```python
from build123d import *

# Parameters (mm, degrees)
BOSS_EXTRUDE1_DEPTH = 28.575
CUT_EXTRUDE1_REACH  = 35.651
SKETCH2_R           = 1.5
CUT_EXTRUDE2_REACH  = 35.651
SKETCH3_R           = 1.5
FILLET1_R           = 2.54


with BuildPart() as part:
    # Sketch1 → Boss-Extrude1 (new body)
    with BuildSketch(Plane.XY):
        Polygon((-1.3335, 11.523094809), (-3.365093559, 11.563734809), (-3.596414524, 0), (3.596414524, 0), (3.365093559, 11.563734809), (1.3335, 11.523094809), (1.524, 2), (-1.524, 2), align=None)
        Polygon((-1.23825, 16.284642214), (-1.3335, 11.523094809), (-3.365093559, 11.563734809), (-3.269843559, 16.325282214), align=None)
    extrude(amount=BOSS_EXTRUDE1_DEPTH)

    # Sketch2 → Cut-Extrude1 (cut, up to next)
    with BuildSketch(Plane(origin=(3.594975959, 0.071913903, 0), x_dir=(0, 0, -1), z_dir=(0.9997999799959991, 0.01999999999999963, 0)), mode=Mode.PRIVATE) as cut_extrude1_sk1:
        with Locations(Location((-23.8125, 8.31911996, 0), (0, 0, 90))):
            Circle(SKETCH2_R)
    cut_extrude1_tool1 = extrude(cut_extrude1_sk1.sketch, amount=-CUT_EXTRUDE1_REACH, mode=Mode.PRIVATE) & part.part
    # Sketch2 → Cut-Extrude1 (cut, up to next)
    with BuildSketch(Plane(origin=(3.594975959, 0.071913903, 0), x_dir=(0, 0, -1), z_dir=(0.9997999799959991, 0.01999999999999963, 0)), mode=Mode.PRIVATE) as cut_extrude1_sk2:
        with Locations(Location((-4.7625, 8.31911996, 0), (0, 0, 90))):
            Circle(SKETCH2_R)
    cut_extrude1_tool2 = extrude(cut_extrude1_sk2.sketch, amount=-CUT_EXTRUDE1_REACH, mode=Mode.PRIVATE) & part.part
    add(cut_extrude1_tool1.solids().sort_by_distance((3.428594, 8.38937, 23.8125))[0], mode=Mode.SUBTRACT)
    add(cut_extrude1_tool2.solids().sort_by_distance((3.428594, 8.38937, 4.7625))[0], mode=Mode.SUBTRACT)

    # Sketch3 → Cut-Extrude2 (cut, up to next)
    with BuildSketch(Plane(origin=(-3.594975959, 0.071913903, 0), x_dir=(0, 0, 1), z_dir=(-0.9997999799959991, 0.019999999999999622, 0)), mode=Mode.PRIVATE) as cut_extrude2_sk1:
        with Locations(Location((4.7625, 8.29879996, 0), (0, 0, 270))):
            Circle(SKETCH3_R)
    cut_extrude2_tool1 = extrude(cut_extrude2_sk1.sketch, amount=-CUT_EXTRUDE2_REACH, mode=Mode.PRIVATE) & part.part
    # Sketch3 → Cut-Extrude2 (cut, up to next)
    with BuildSketch(Plane(origin=(-3.594975959, 0.071913903, 0), x_dir=(0, 0, 1), z_dir=(-0.9997999799959991, 0.019999999999999622, 0)), mode=Mode.PRIVATE) as cut_extrude2_sk2:
        with Locations(Location((23.8125, 8.29879996, 0), (0, 0, 270))):
            Circle(SKETCH3_R)
    cut_extrude2_tool2 = extrude(cut_extrude2_sk2.sketch, amount=-CUT_EXTRUDE2_REACH, mode=Mode.PRIVATE) & part.part
    add(cut_extrude2_tool1.solids().sort_by_distance((-3.429, 8.369054, 4.7625))[0], mode=Mode.SUBTRACT)
    add(cut_extrude2_tool2.solids().sort_by_distance((-3.429, 8.369054, 23.8125))[0], mode=Mode.SUBTRACT)

    # Fillet1
    # the kernel refuses this fillet: 2.54 mm, written as the material it takes off along each edge
    with BuildSketch(Plane(origin=(1.3335, 11.523094809, -6.221703947), x_dir=(0.9997999799960309, 0.019999999998416385, 0), z_dir=(0, 0, 1))) as fillet1_piece_1:
        with BuildLine():
            CenterArc((2.54, -2.488681579), FILLET1_R, 101.536959033, 78.463040967)
            Line((0, -2.488681579), (-0.0508, -2.488681579))
            Line((-0.0508, -2.488681579), (-0.0508, 0))
            Line((-0.0508, 0), (0, 0.0508))
            ThreePointArc((0, 0.0508), (1.016, 0.0508), (2.02184, 0.049773632))
            Line((2.02184, 0.049773632), (2.032, 0))
        make_face()
    extrude(amount=41.018407893, mode=Mode.SUBTRACT)
    with BuildSketch(Plane(origin=(-1.23825, 16.284642214, -6.221703947), x_dir=(-0.9997999799960307, 0.019999999998425156, 0), z_dir=(0, 0, 1))) as fillet1_piece_2:
        with BuildLine():
            CenterArc((2.54, 2.488681579), FILLET1_R, 180, 78.463040967)
            Line((0, 2.488681579), (-0.0508, 2.488681579))
            Line((-0.0508, 2.488681579), (-0.0508, 0))
            Line((-0.0508, 0), (0, -0.0508))
            ThreePointArc((0, -0.0508), (1.016, -0.0508), (2.02184, -0.049773632))
            Line((2.02184, -0.049773632), (2.032, 0))
        make_face()
    extrude(amount=41.018407893, mode=Mode.SUBTRACT)


solid = part.part
```
The model under review builds one solid part; all positions refer to its coordinate system, in mm. A direction names the side the tool comes from. Round coordinates to 2 decimals unless told otherwise and drop trailing zeros. Loops run counter-clockwise (first coordinate to the right, second up) from the corner with the lowest first, then second, coordinate; pieces in that order, holes last. Notation, with made-up numbers: (-3.75, -4.75) - (39.25, -4.75) arc R30 ccw to (39.25, 31.25) - close; hole circle Ø11 at (68.5, 49.25). An arc over 180 degrees is marked (long way). Use a Markdown table: item, result. Add a question column.
Q1. Machinability: for faces 1 (the face through (-2, 6, 28.575)), 2 (the face through (-2.42, 8.54, 25.3)), which of the approach directions +Z, -Z, +X, -X, +Y, -Y give a long, thin tool a straight path to every point of the face, cutting with its end or side? Answer none if there is none.
Q2. Add section D-D (x = 2). State how many separate pieces and enclosed holes the cut face has, plus the area to 3 significant figures.
Q3. Add section C-C (z = 15.5). State the section outline as (x, y) points, plus the area to 3 significant figures.
Q4. Add section B-B (y = 3.5). State the section outline as (x, z) points (3 decimals).
Q5. The part is to be moulded in two halves that separate along Y. For faces 3 (the face through (-2.421, 8.674, 3.298)), 4 (the face through (0, 0, 14)), 5 (the face through (-2, 6, 0)), say which applies: pulls with the +Y half, pulls with the -Y half, needs draft (parallel to the pull), parting line crosses it, or undercut.
Q6. Insertion check: pin 1 Ø2.5 at (x, z) = (-0.5, 17.5) entering from +Y; pin 2 Ø1.5 at (x, y) = (1.5, 11.5) entering from +Z; pin 3 Ø2 at (x, z) = (1.5, 8) entering from +Y. Each pin has a flat end and moves straight along its axis. Give the tip position at first contact, or say it passes through.
Q7. For probe 1 along Z at (x, y) = (2.25, 8.5) (3 decimals); probe 2 along Y at (x, z) = (-0.75, 9.25); probe 3 along X at (y, z) = (10.25, 14), list the stretches that pass through material, from the lowest coordinate up.
Q8. Add section A-A (z = 4). State the section outline as (x, y) points.
Worked answers:
| question | item | result |
|---|---|---|
| 1 | face 1 | +Z, +X, -X, +Y, -Y |
| 1 | face 2 | none |
| 2 | separate pieces | 1 |
| 2 | enclosed holes | 2 |
| 2 | area | 293 mm² |
| 3 | outline | (-3.6, 0) - (3.6, 0) - (3.37, 11.56) arc R2.54 ccw to (1.38, 9.03) - (1.52, 2) - (-1.52, 2) - (-1.29, 13.8) arc R2.54 ccw to (-3.27, 16.33) - close |
| 3 | area | 60.2 mm² |
| 4 | outline | (-3.526, 0) - (-1.494, 0) - (-1.494, 28.575) - (-3.526, 28.575) - close; (1.494, 0) - (3.526, 0) - (3.526, 28.575) - (1.494, 28.575) - close |
| 5 | face 3 | undercut |
| 5 | face 4 | pulls with the -Y half |
| 5 | face 5 | needs draft |
| 6 | pin 1 | y = 15.31 |
| 6 | pin 2 | through |
| 6 | pin 3 | y = 11.19 |
| 7 | probe 1 | 0 to 3.269, 6.256 to 22.319, 25.306 to 28.575 |
| 7 | probe 2 | 0 to 2 |
| 7 | probe 3 | -3.39 to -1.36, 1.67 to 3.39 |
| 8 | outline | (-3.6, 0) - (3.6, 0) - (3.45, 7.1) - (1.42, 7.06) - (1.52, 2) - (-1.52, 2) - (-1.42, 7.04) - (-3.45, 7.08) - close; (-3.4, 9.66) - (-1.37, 9.62) - (-1.29, 13.8) arc R2.54 ccw to (-3.27, 16.33) - close; (1.44, 9.64) - (3.4, 9.68) - (3.37, 11.56) arc R2.54 ccw to start |
